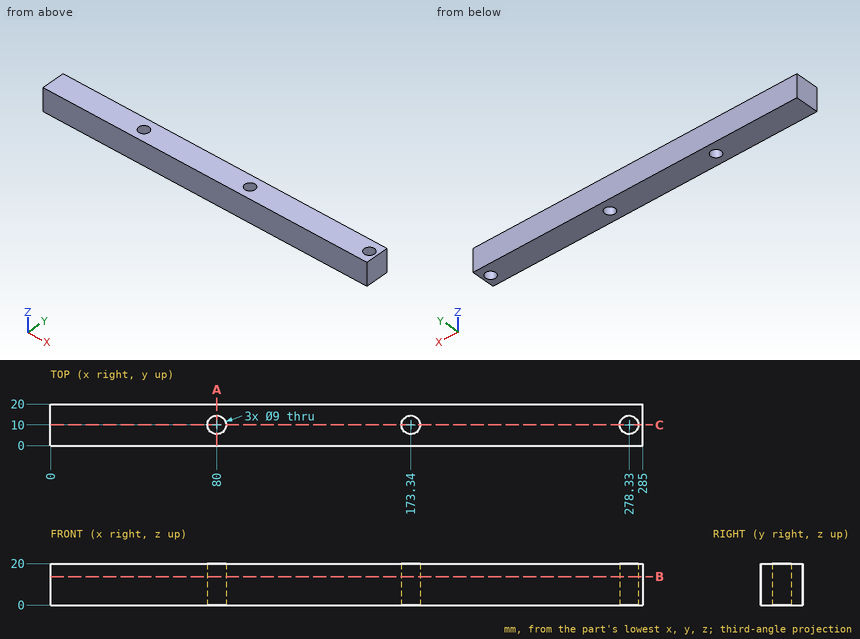
Input: dimensioned drawing with shaded views. Units: mm. Origin: part minimum x, y, z. Coordinates: 2 decimals unless noted, no trailing zeros. Write each loop counter-clockwise with the first axis right and the second up, starting at its lowest first coordinate (ties: lowest second). Pieces come first, ordered by that corner, then holes. Notation, with made-up numbers: (68, -7) -> (107, -7) arc R24 ccw to (107, 11) -> close; hole circle Ø1 at (42.5, 67). An arc over 180 degrees is marked (long way). Return JSON: item names as keys, results as strings. Group by question number.
1) Section query C-C, the plane y = 10. Return loops of the section in (x, z), plus the area to 3 significant figures.
2) Ray query, line 1 along X through (y, z) = (10.25, 7.75); line 2 along Y through (x, z) = (173.34, 5.75); line 3 along X through (y, z) = (10.5, 7.5). Return the intervals inside material, ascending.
3) Section query A-A, the plane x = 80. Return loops of the section in (y, z), plus the area to 3 significant figures.
4) Section query B-B, the plane z = 13.75. Return loops of the section in (x, y).
From the geometry:
{
 "1": {"outline": "(0, 0) -> (75.5, 0) -> (75.5, 20) -> (0, 20) -> close; (84.5, 0) -> (168.84, 0) -> (168.84, 20) -> (84.5, 20) -> close; (177.84, 0) -> (273.83, 0) -> (273.83, 20) -> (177.84, 20) -> close; (282.83, 0) -> (285, 0) -> (285, 20) -> (282.83, 20) -> close", "area": "5,160 mm²"},
 "2": {"line 1": "0 to 75.51, 84.49 to 168.85, 177.83 to 273.84, 282.82 to 285", "line 2": "0 to 5.5, 14.5 to 20", "line 3": "0 to 75.53, 84.47 to 168.87, 177.81 to 273.86, 282.8 to 285"},
 "3": {"outline": "(0, 0) -> (5.5, 0) -> (5.5, 20) -> (0, 20) -> close; (14.5, 0) -> (20, 0) -> (20, 20) -> (14.5, 20) -> close", "area": "220 mm²"},
 "4": {"outline": "(0, 0) -> (285, 0) -> (285, 20) -> (0, 20) -> close; hole circle Ø9 at (80, 10); hole circle Ø9 at (173.34, 10); hole circle Ø9 at (278.33, 10)"}
}
